```python
from build123d import *

# Parameters (mm, degrees)
EXTRUDE_1_DEPTH     = 10
SKETCH_2_R          = 6.5
CUT_EXTRUDE_1_DEPTH = 10
CUT_EXTRUDE_2_DEPTH = 10
FILLET_1_R          = 1
EXTRUDE_START       = -10
EXTRUDE_2_DEPTH     = 10
SKETCH_5_R          = 1.55
SKETCH_5_R_2        = 2.05
CUT_EXTRUDE_3_DEPTH = 10
SKETCH_6_R          = 11.5
CUT_EXTRUDE_4_DEPTH = 10


with BuildPart() as part:
    # 草图1 → 凸台-拉伸1 (new body)
    with BuildSketch(Plane.XY):
        with BuildLine():
            Line((200.1875, 14.998828079), (0.21875, 17.498632759))
            ThreePointArc((0.21875, 17.498632759), (-17.5, 0), (0.21875, -17.498632759))
            Line((0.21875, -17.498632759), (200.1875, -14.998828079))
            ThreePointArc((200.1875, -14.998828079), (215, 0), (200.1875, 14.998828079))
        make_face()
    extrude(amount=EXTRUDE_1_DEPTH)

    # 草图2 → 切除-拉伸1 (cut)
    with BuildSketch(Plane.XY.offset(10)):
        Circle(SKETCH_2_R)
    extrude(amount=-CUT_EXTRUDE_1_DEPTH, mode=Mode.SUBTRACT)

    # 草图3 → 切除-拉伸2 (cut)
    with BuildSketch(Plane.XY.offset(10)):
        Polygon((24.289001935, 12.19734043), (85.658139631, 11.430166271), (16.937408094, -6.979422532), align=None)
        Polygon((16.414613885, -12.295777972), (84.346077325, 5.902373893), (91.781134838, -11.353622851), align=None)
        Polygon((106.93275646, -6.06439659), (114.284350301, 13.112366373), (175.653487997, 12.345192214), align=None)
        Polygon((181.776483204, -10.438596909), (106.409962251, -11.380752029), (174.341425691, 6.817399835), align=None)
    extrude(amount=-CUT_EXTRUDE_2_DEPTH, mode=Mode.SUBTRACT)

    # 圆角1
    fillet_1_edges = [part.edges().sort_by_distance(p)[0] for p in [
        (84.346077325, 5.902373893, 5),
        (91.781134838, -11.353622851, 5),
        (16.414613885, -12.295777972, 5),
        (175.653487997, 12.345192214, 5),
        (106.93275646, -6.06439659, 5),
        (114.284350301, 13.112366373, 5),
        (174.341425691, 6.817399835, 5),
        (181.776483204, -10.438596909, 5),
        (106.409962251, -11.380752029, 5),
        (85.658139631, 11.430166271, 5),
        (16.937408094, -6.979422532, 5),
        (24.289001935, 12.19734043, 5),
    ]]
    fillet(fillet_1_edges, radius=FILLET_1_R)

    # 草图4 → 凸台-拉伸2 (add)
    with BuildSketch(Plane.XY.offset(10).offset(EXTRUDE_START)):
        with BuildLine():
            Line((186.959776982, 15.164187536), (200.1875, 14.998828079))
            ThreePointArc((200.1875, 14.998828079), (215, 0), (200.1875, -14.998828079))
            Line((200.1875, -14.998828079), (186.959776982, -15.164187536))
            ThreePointArc((186.959776982, -15.164187536), (220, 0), (186.959776982, 15.164187536))
        make_face()
    extrude(amount=EXTRUDE_2_DEPTH)

    # 草图5 → 切除-拉伸3 (cut)
    with BuildSketch(Plane.XY.offset(10)):
        with Locations((200, 15)):
            Circle(SKETCH_5_R)
        with Locations((215, 0)):
            Circle(SKETCH_5_R)
        with Locations((200, -15)):
            Circle(SKETCH_5_R)
        with Locations((185, 0)):
            Circle(SKETCH_5_R)
        with Locations((189.393398282, 10.606601718)):
            Circle(SKETCH_5_R_2)
        with Locations((210.606601718, 10.606601718)):
            Circle(SKETCH_5_R_2)
        with Locations((210.606601718, -10.606601718)):
            Circle(SKETCH_5_R_2)
        with Locations((189.393398282, -10.606601718)):
            Circle(SKETCH_5_R_2)
    extrude(amount=-CUT_EXTRUDE_3_DEPTH, mode=Mode.SUBTRACT)

    # 草图6 → 切除-拉伸4 (cut)
    with BuildSketch(Plane.XY.offset(10)):
        with Locations((200, 0)):
            Circle(SKETCH_6_R)
    extrude(amount=-CUT_EXTRUDE_4_DEPTH, mode=Mode.SUBTRACT)


solid = part.part
```
Part model, mm, in its own coordinate system. A direction names the side the tool comes from. Round coordinates to 2 decimals unless told otherwise and drop trailing zeros. Use CSV: the item, a comma, the result in double quotes. Start each with the question number.
1) Wall check: L1, parallel to Y at x = 200, z = 6; L2, parallel to Y at x = 58.5, z = 8.75; L3, parallel to Y at x = 158, z = 5.75. Give the ranges that are in metal, low to high. Write a range as [from, to].
2) Cut at A-A, the plane z = 2.75. Give the number of separate pieces and of enclosed holes in the cut face, plus the area to 3 significant figures.
3) Which spindle directions (+Z, -Z, +X, -X, +Y, -Y) get a long thin tool onto all of the face, cutting with end or side? Do faces 4 (the flat face through (100, 0, 10)), 5 (the flat face through (177.888, -1.414, 5.07)). Say none if no direction does.
4) Drop flat-ended pins along their axis: P1, Ø2, axis at x = 104.5, z = 9, coming from the +Y side; P2, Ø4, axis at x = 118, z = 5.5, coming from the -Y side. Give the stop position or say it passes through.
5) Pull direction Y, two halves, no side cores. Call faces 1 (the cylindrical face through (219.99, -0.64, 4.93)), 2 (the flat face through (100, 0, 0)), 3 (the flat face through (143.4, -1.47, 5.07)): +Y half, -Y half, draft (parallel to the pull), parting line (faces both ways), or undercut.
Determined:
1,L1,"y = [-20, -16.55], [-13.45, -11.5], [11.5, 13.45], [16.55, 20]"
1,L2,"y = [-16.77, -11.77], [-1.02, 4.15], [11.77, 16.77]"
1,L3,"y = [-15.53, -10.74], [2.44, 7.62], [12.57, 15.53]"
2,separate pieces,"1"
2,enclosed holes,"14"
2,area,"4,610 mm2"
3,face 4,"+Z, +X, -X, +Y, -Y"
3,face 5,"+Z, -Z"
4,P1,"stops at y = 16.21"
4,P2,"stops at y = -16.05"
5,face 1,"parting line"
5,face 2,"draft"
5,face 3,"undercut"
